Source: CAD feature listing. Evaluate the final solid. Frame: model axes, mm. A direction names the side the tool comes from. Round coordinates to 2 decimals unless told otherwise and drop trailing zeros. Loops run counter-clockwise (first coordinate to the right, second up) from the corner with the lowest first, then second, coordinate; pieces in that order, holes last. Notation, with made-up numbers: (-37, 56) -> (-20, 56) arc R23 ccw to (-20, 65) -> close; hole circle Ø5 at (60, 55). An arc over 180 degrees is marked (long way). Write item = value, one per line.
from build123d import *

# Parameters (mm, degrees)
SKETCH_1_R      = 1.5
SKETCH_1_R_2    = 2
SKETCH_1_W      = 4
SKETCH_1_H      = 10
EXTRUDE_1_DEPTH = 2
FILLET_1_R      = 1


with BuildPart() as part:
    # Эскиз1 → Бобышка-Вытянуть1 (new body)
    with BuildSketch(Plane(origin=(0, 0, 0), x_dir=(1, 0, 0), z_dir=(0, 1, 0))):
        with BuildLine():
            Line((-2, 30), (48.3, 30))
            Line((48.3, 30), (75.8, 27))
            ThreePointArc((75.8, 27), (87.8, 15), (75.8, 3))
            Line((75.8, 3), (48.3, 0))
            Line((48.3, 0), (-2, 0))
            Line((-2, 0), (-2, 30))
        make_face()
        with Locations(Location((3.4, 10, 0), (0, 0, 270))):
            Circle(SKETCH_1_R, mode=Mode.SUBTRACT)
        with Locations(Location((3.4, 20, 0), (0, 0, 270))):
            Circle(SKETCH_1_R, mode=Mode.SUBTRACT)
        with Locations(Location((52.6, 10, 0), (0, 0, 270))):
            Circle(SKETCH_1_R, mode=Mode.SUBTRACT)
        with Locations(Location((52.6, 20, 0), (0, 0, 270))):
            Circle(SKETCH_1_R, mode=Mode.SUBTRACT)
        with Locations(Location((75.8, 15, 0), (0, 0, 270))):
            Circle(SKETCH_1_R_2, mode=Mode.SUBTRACT)
        Polygon((8, 25.5), (48.3, 25.5), (48.3, 16), (56.3, 16), (56.3, 14), (48.3, 14), (48.3, 4.5), (8, 4.5), (8, 14), (0, 14), (0, 16), (8, 16), align=None, mode=Mode.SUBTRACT)
        with Locations((63.3, 15)):
            Rectangle(SKETCH_1_W, SKETCH_1_H, mode=Mode.SUBTRACT)
    extrude(amount=EXTRUDE_1_DEPTH)

    # Скругление1
    fillet_1_edges = [part.edges().sort_by_distance(p)[0] for p in [
        (65.3, 1, -10),
        (65.3, 1, -20),
        (61.3, 1, -20),
        (61.3, 1, -10),
    ]]
    fillet(fillet_1_edges, radius=FILLET_1_R)


solid = part.part
1. Set-up query: faces 1 (the face through (54, 0, -12)), 2 (the face through (4, 1, -14)). Return all of +Z, -Z, +X, -X, +Y, -Y with unobstructed straight access to the full face (end or side cutting, diameter ignored); none if empty.
Evaluation:
face_1 = +Z, -Z, +X, -X, -Y
face_2 = +Y, -Y
2. Mould query, pull axis Z, two halves, no side actions, for faces 3 (the face through (87.797, 0.986, -15.264)), 4 (the face through (28, 1, -4.5)), 5 (the face through (-2, 1, -15)), 6 (the face through (4, 1, -16)). Classes: released by +Z, released by -Z, zero draft, split by the parting line, or undercut.
Evaluation:
face_3 = split by the parting line
face_4 = undercut
face_5 = zero draft
face_6 = undercut
3. Section query C-C (x = 35). Return the cut outline in (y, z), then the cut area to 3 significant figures.
Evaluation:
outline = (0, -30) -> (2, -30) -> (2, -25.5) -> (0, -25.5) -> close; (0, -4.5) -> (2, -4.5) -> (2, 0) -> (0, 0) -> close
area = 18.0 mm²
4. Section query D-D (y = 1.05). Give the number of separate pieces and of enclosed holes in the cut face, then the cut area to 3 significant figures.
Evaluation:
separate_pieces = 1
enclosed_holes = 7
area = 1,520 mm²
5. Section query A-A (z = -15). Return the cut outline in (x, y), then the cut area to 3 significant figures.
Evaluation:
outline = (-2, 0) -> (0, 0) -> (0, 2) -> (-2, 2) -> close; (56.3, 0) -> (61.3, 0) -> (61.3, 2) -> (56.3, 2) -> close; (65.3, 0) -> (73.8, 0) -> (73.8, 2) -> (65.3, 2) -> close; (77.8, 0) -> (87.8, 0) -> (87.8, 2) -> (77.8, 2) -> close
area = 51.0 mm²
6. Section query B-B (x = 3.4). Return the cut outline in (y, z), then the cut area to 3 significant figures.
Evaluation:
outline = (0, -30) -> (2, -30) -> (2, -21.5) -> (0, -21.5) -> close; (0, -18.5) -> (2, -18.5) -> (2, -16) -> (0, -16) -> close; (0, -14) -> (2, -14) -> (2, -11.5) -> (0, -11.5) -> close; (0, -8.5) -> (2, -8.5) -> (2, 0) -> (0, 0) -> close
area = 44.0 mm²
7. Line query: probe 1 along X at (y, z) = (0.65, -15); probe 2 along Z at (x, y) = (15.5, 0.15); probe 3 along X at (y, z) = (1.5, -14.5). Output: solid intervals per line, ascending. Write a range as from..to.
Evaluation:
probe_1 = -2..0, 56.3..61.3, 65.3..73.8, 77.8..87.8
probe_2 = -30..-25.5, -4.5..0
probe_3 = -2..0, 56.3..61.3, 65.3..73.86, 77.74..87.79
8. Contact query for a flat-ended pin moving along its axis: pin 1 Ø0.6 at (y, z) = (1.5, -16.5) entering from +X. Output: stop coordinate, or through.
Evaluation:
pin_1 = 87.74
